Verification items for the finished model (mm, model axes). Face numbers are marked on the shaded views. Coordinates: 2 decimals unless noted, no trailing zeros. Order: outer loops, then holes, each group sorted by start corner. A loop starts at its lowest first (then second) coordinate and runs counter-clockwise, first axis right, second up. Notation, with made-up numbers: M -18,83 L 15,83 A9 ccw 15,91 Z; hole C -3.75,20 d4. An arc over 180 degrees is marked long. Return JSON: item names as keys, results as strings.
```python
from build123d import *

# Parameters (mm, degrees)
SKETCH_W        = 175
SKETCH_H        = 100
PAD_DEPTH       = 5
FILLET_R        = 10
SKETCH001_R     = 3.4
SKETCH001_W     = 16
SKETCH001_H     = 16
POCKET_DEPTH    = 5.001
SKETCH002_W     = 189.697797
SKETCH002_H     = 117.830608
POCKET001_DEPTH = 2
SKETCH003_W     = 43.44
SKETCH003_H     = 41.15
POCKET002_DEPTH = 4.5
SKETCH004_R     = 3
POCKET003_DEPTH = 3


with BuildPart() as part:
    # Sketch → Pad (new body)
    with BuildSketch(Plane.XY):
        with Locations((-10.270103, -10.695957)):
            Rectangle(SKETCH_W, SKETCH_H)
    extrude(amount=PAD_DEPTH)

    # Fillet
    fillet_edges = [part.edges().sort_by_distance(p)[0] for p in [
        (-97.770103, -60.695957, 2.5),
        (-97.770103, 39.304043, 2.5),
        (77.229897, -60.695957, 2.5),
        (77.229897, 39.304043, 2.5),
    ]]
    fillet(fillet_edges, radius=FILLET_R)

    # Sketch001 → Pocket (cut, through all)
    with BuildSketch(Plane.XY.offset(5)):
        with Locations((-73, 0)):
            Circle(SKETCH001_R)
        with Locations((-26, -45)):
            Rectangle(SKETCH001_W, SKETCH001_H)
        with Locations((0, -45)):
            Rectangle(SKETCH001_W, SKETCH001_H)
        with Locations((26, -45)):
            Rectangle(SKETCH001_W, SKETCH001_H)
        with Locations((61, 13)):
            Rectangle(SKETCH001_W, SKETCH001_H)
        with Locations((61, -13)):
            Rectangle(SKETCH001_W, SKETCH001_H)
    extrude(amount=-POCKET_DEPTH, mode=Mode.SUBTRACT)

    # Sketch002 → Pocket001 (cut)
    with BuildSketch(Plane(origin=(0, 0, 0), x_dir=(1, 0, 0), z_dir=(0, 0, -1))):
        with Locations((-11.809575, 11.293159)):
            Rectangle(SKETCH002_W, SKETCH002_H)
        with BuildLine():
            Line((-87.770101, 56.695957), (67.229895, 56.695957))
            ThreePointArc((73.229897, 50.695985), (71.472527, 54.938608), (67.229895, 56.695957))
            Line((73.229897, 50.695985), (73.229897, -29.304043))
            ThreePointArc((67.229897, -35.304043), (71.472538, -33.546684), (73.229897, -29.304043))
            Line((-87.770103, -35.304043), (67.229897, -35.304043))
            ThreePointArc((-93.770103, -29.304043), (-92.012744, -33.546684), (-87.770103, -35.304043))
            Line((-93.770103, 50.695985), (-93.770103, -29.304043))
            ThreePointArc((-87.770101, 56.695957), (-92.012733, 54.938608), (-93.770103, 50.695985))
        make_face(mode=Mode.SUBTRACT)
    extrude(amount=-POCKET001_DEPTH, mode=Mode.SUBTRACT)

    # Sketch003 → Pocket002 (cut)
    with BuildSketch(Plane(origin=(0, 0, 0), x_dir=(1, 0, 0), z_dir=(0, 0, -1))):
        Rectangle(SKETCH003_W, SKETCH003_H)
    extrude(amount=-POCKET002_DEPTH, mode=Mode.SUBTRACT)

    # Sketch004 → Pocket003 (cut)
    with BuildSketch(Plane(origin=(0, 0, 0), x_dir=(1, 0, 0), z_dir=(0, 0, -1))):
        with Locations((-34, 45)):
            Circle(SKETCH004_R)
        with Locations((-18, 45)):
            Circle(SKETCH004_R)
        with Locations((-8, 45)):
            Circle(SKETCH004_R)
        with Locations((8, 45)):
            Circle(SKETCH004_R)
        with Locations((18, 45)):
            Circle(SKETCH004_R)
        with Locations((34, 45)):
            Circle(SKETCH004_R)
        with Locations((61, 21)):
            Circle(SKETCH004_R)
        with Locations((61, 5)):
            Circle(SKETCH004_R)
        with Locations((61, -5)):
            Circle(SKETCH004_R)
        with Locations((61, -21)):
            Circle(SKETCH004_R)
    extrude(amount=-POCKET003_DEPTH, mode=Mode.SUBTRACT)


solid = part.part
```
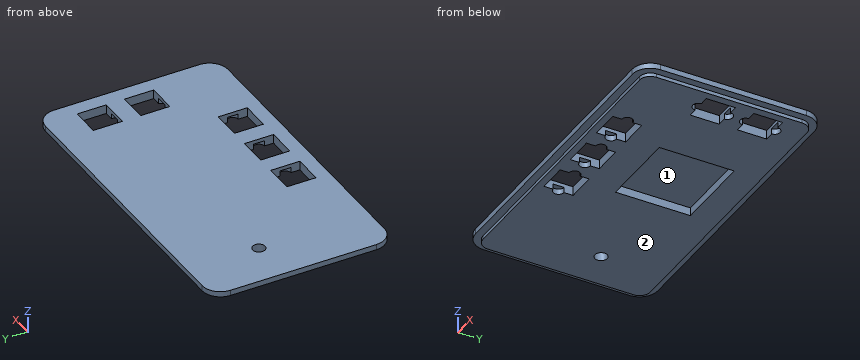
Q1. Cross-section at A-A, the plane y = -45. State how many separate pieces and enclosed holes the cut face has, and give its area (3 significant figures).
Values:
{"separate pieces": "4", "enclosed holes": "0", "area": "565 mm^2"}
Q2. Go/stop test with flat-tipped pins: pin 1 (1 mm diameter, centred on y = -3.5, z = 1, fed in from -X); pin 2 (3.5 mm diameter, centred on x = -17, y = -45.5, fed in from -Z); pin 3 (20.5 mm diameter, centred on x = -4, y = -5, fed in from -Z). Record where each tip stops, or that it passes through.
Values:
{"pin 1": "x = -93.77", "pin 2": "z = 3", "pin 3": "z = 4.5"}
Q3. Cross-section at C-C, the plane y = 0. Record the boundary of the cut face in (x, z), and give its area (3 significant figures).
Values:
{"outline": "M -97.77,2 L -93.77,2 L -93.77,0 L -76.4,0 L -76.4,5 L -97.77,5 Z; M -69.6,0 L -21.72,0 L -21.72,4.5 L 21.72,4.5 L 21.72,0 L 73.23,0 L 73.23,2 L 77.23,2 L 77.23,5 L -69.6,5 Z", "area": "630 mm^2"}
Q4. Draft check along X on the marked faces 1 and 2. Enter one of: pulls with the +X half, pulls with the -X half, needs draft (parallel to the pull), parting line crosses it, or undercut.
Values:
{"face 1": "undercut", "face 2": "needs draft"}
Q5. Material ranges on line 1 along X through (y, z) = (-16, 3.95); line 2 along X through (y, z) = (-12.5, 1.4); line 3 along X through (y, z) = (-50.5, 3.6), recorded low to high.
Values:
{"line 1": "-97.77 to -21.72, 21.72 to 53, 69 to 77.23", "line 2": "-93.77 to -21.72, 21.72 to 53, 69 to 73.23", "line 3": "-97.77 to -34, -18 to -8, 8 to 18, 34 to 77.23"}
Q6. Cross-section at B-B, the plane x = -25.5. Record the boundary of the cut face in (y, z), and give its area (3 significant figures).
Values:
{"outline": "M -60.7,2 L -56.7,2 L -56.7,0 L -53,0 L -53,5 L -60.7,5 Z; M -37,0 L 35.3,0 L 35.3,2 L 39.3,2 L 39.3,5 L -37,5 Z", "area": "404 mm^2"}
Q7. Cross-section at D-D, the plane x = 61. Record the boundary of the cut face in (y, z).
Values:
{"outline": "M -60.7,2 L -56.7,2 L -56.7,0 L -24,0 L -24,3 L -21,3 L -21,5 L -60.7,5 Z; M -5,3 L -2,3 L -2,0 L 2,0 L 2,3 L 5,3 L 5,5 L -5,5 Z; M 21,3 L 24,3 L 24,0 L 35.3,0 L 35.3,2 L 39.3,2 L 39.3,5 L 21,5 Z"}
